Could you check a few things on this model? Use its own coordinates, in mm. A direction names the side the tool comes from. Round coordinates to 2 decimals unless told otherwise and drop trailing zeros. Loops run counter-clockwise (first coordinate to the right, second up) from the corner with the lowest first, then second, coordinate; pieces in that order, holes last. Notation, with made-up numbers: M 31,85 L 47,85 A22 ccw 47,94 Z; hole C 0,44.25 d10. An arc over 180 degrees is marked long. One line per item, written item: value. Start each with the question number.
Q1. Please list where these lines run through material, in increasing order: line 1 along Z through (x, y) = (-40, 3.7); line 2 along Y through (x, z) = (-40.5, -67.5); line 3 along Z through (x, y) = (-7.5, 29).
Q2. Which directions (+Z, -Z, +X, -X, +Y, -Y) give clear straight access to the entire face, cutting with the end or side of a thin tool? Please do faces 1 (the face through (-15, 65, -75)), 2 (the face through (-43, 7, -71)), 3 (the face through (-25, 5, -29)).
Q3. Thinking about a two-plate mould opening in Z: for faces 4 (the face through (-40.066, 41.048, -65.07)), 5 (the face through (-7, 6, -72)), 6 (the face through (-10, 2, -102)), which applies, released by +Z, released by -Z, zero draft, split by the parting line, or undercut?
Q4. Imagine slicing it at B-B (z = -10). Please give me the cut outline in (x, y).
Q5. Imagine slicing it at A-A (y = 16). Please give me the cut outline in (x, z).
Q6. I'm going to push flat-ended pins straight in: pin 1 Ø4 at (x, y) = (-8, 24) entering from +Z; pin 2 Ø5 at (x, z) = (-28.5, -50.5) entering from +Y; pin 3 Ø8 at (y, z) = (93, -75.5) entering from +X; pin 4 Ø5.5 at (x, z) = (-24, -80) entering from +Y. Where does each tip first touch, or does it pass through?
Q7. Imagine slicing it at D-D (x = -45.5). Please give me the cut outline in (y, z), then the cut area to 3 significant figures.
Q8. Imagine slicing it at C-C (x = -9.5). Please give me the cut outline in (y, z).
Autodesk Inventor part; units mm, degrees
ref_plane "YZ Plane" through (0, 0, 0) normal (1, 0, 0) x (0, 1, 0)
ref_plane "XZ Plane" through (0, 0, 0) normal (0, 1, 0) x (-1, 0, 0)
ref_plane "XY Plane" through (0, 0, 0) normal (0, 0, 1) x (1, 0, 0)
sketch "Sketch1" plane through (0, 0, 0) normal (0, 1, 0) x (-1, 0, 0)
  point P0 (0, 0)
sketch "Sketch2" plane through (0, 0, 0) normal (0, 1, 0) x (-1, 0, 0)
  line L0 (0, 0) -> (50, 0)
  line L1 (50, 0) -> (50, -110)
  line L2 (50, -110) -> (0, -110)
  line L3 (0, -110) -> (0, 0)
  line L4 (25, 0) -> (25, -110) construction
  line L5 (50, -55) -> (0, -55) construction
  circle A0 centre (40, -10) radius 2
  circle A1 centre (40, -100) radius 2
  circle A2 centre (10, -10) radius 2
  circle A3 centre (10, -100) radius 2
  dimension "d0" = 50
  dimension "d1" = 110
  dimension "d2" = 4
  dimension "d3" = 10
  dimension "d4" = 10
  dimension "d7" = 90
  dimension "d10" = 30
extrude "Extrusion1" add sketch "Sketch2" along normal blind 5
sketch "Sketch3" plane through (0, 5, 0) normal (0, 1, 0) x (1, 0, 0)
  line L0 (-50, 110) -> (-50, 0)
  line L1 (0, 60) -> (-50, 60)
  line L2 (-50, 60) -> (-50, 70)
  line L3 (0, 70) -> (0, 60)
  line L4 (-50, 0) -> (0, 0)
  line L5 (0, 110) -> (-50, 110) construction
  line L6 (0, 0) -> (0, 110)
  circle A0 centre (-25, 80) radius 3.5
  arc A1 (-15, 80) -> (-35, 80) centre (-25, 80) ccw
  line L7 (-35, 80) -> (-35, 70)
  line L8 (-15, 80) -> (-15, 70)
  line L9 (-50, 70) -> (-35, 70)
  line L10 (-15, 70) -> (0, 70)
  dimension "d15" = 60
  dimension "d17" = 7
  dimension "d18" = 30
extrude "Extrusion2" add sketch "Sketch3" along normal blind 120 contours L9 L7 A1 L8 L10 L3 L1 L0
chamfer "Chamfer1" distance 2 angle 45 1 edges at (-25, 5, -60)
chamfer "Chamfer2" distance 3 angle 45 5 edges at (-7.5, 5, -70) (-42.5, 5, -70) (-25, 5, -90) (-15, 5, -75) (-35, 5, -75)
sketch "Sketch4" plane through (0, 125, -70) normal (0, 0, -1) x (-1, 0, 0)
  line L0 (0, 0) -> (15, 0)
  line L1 (15, -117) -> (0, -117)
  line L2 (35, 0) -> (50, 0)
  line L3 (50, -117) -> (35, -117)
  circle A0 centre (9.5, -109) radius 2
  circle A1 centre (40.5, -109) radius 2
  circle A2 centre (9.5, -82) radius 2
  circle A3 centre (40.5, -82) radius 2
  line L4 (0, -117) -> (0, 0)
  line L5 (50, -117) -> (50, 0)
  line L6 (0, -120) -> (50, -120)
  point P0 (0, -125)
  dimension "d27" = 4
  dimension "d29" = 4
  dimension "d31" = 4
  dimension "d32" = 4
  dimension "d33" = 27
  dimension "d34" = 27
  dimension "d35" = 9.5
  dimension "d36" = 9.5
  dimension "d37" = 9.5
  dimension "d38" = 9.5
  dimension "d40" = 11
  dimension "d41" = 11
extrude "Extrusion3" cut sketch "Sketch4" against normal blind 10
chamfer "Chamfer3" distance 2 angle 45 8 edges at (-25, 125, -90) (-35, 125, -75) (-15, 125, -75) (-7.5, 125, -70) (0, 125, -65) (-25, 125, -60) (-42.5, 125, -70) (-50, 125, -65)
chamfer "Chamfer4" distance 3 angle 45 4 edges at (0, 2.5, -110) (-50, 2.5, -110) (0, 2.5, 0) (-50, 2.5, 0)
Report:
1. line 1: z = -110 to -102, -98 to -12, -8 to 0
1. line 2: y = 0 to 14, 18 to 41, 45 to 125
1. line 3: z = -70 to -60
2. face 1: -Z, +X, +Y
2. face 2: -Z, -X, +Y
2. face 3: +Z, +X, -X, +Y
3. face 4: zero draft
3. face 5: released by -Z
3. face 6: undercut
4. outline: M -50,0 L -42,0 L -42,5 L -50,5 Z; M -38,0 L -12,0 L -12,5 L -38,5 Z; M -8,0 L 0,0 L 0,5 L -8,5 Z
5. outline: M -50,-70 L -42.5,-70 L -42.5,-60 L -50,-60 Z; M -38.5,-70 L -35,-70 L -35,-80 A10 ccw -15,-80 L -15,-70 L -11.5,-70 L -11.5,-60 L -38.5,-60 Z; M -7.5,-70 L 0,-70 L 0,-60 L -7.5,-60 Z; hole C -25,-80 d7
6. pin 1: stops at z = -60
6. pin 2: stops at y = 5
6. pin 3: stops at x = -15
6. pin 4: stops at y = 125
7. outline: M 0,-110 L 5,-110 L 5,-73 L 8,-70 L 123,-70 L 125,-68 L 125,-62 L 123,-60 L 7,-60 L 5,-58 L 5,0 L 0,0 Z
7. area: 1,750 mm²
8. outline: M 0,-110 L 5,-110 L 5,-101.94 L 0,-101.94 Z; M 0,-98.06 L 5,-98.06 L 5,-73 L 8,-70 L 14,-70 L 14,-60 L 7,-60 L 5,-58 L 5,-11.94 L 0,-11.94 Z; M 0,-8.06 L 5,-8.06 L 5,0 L 0,0 Z; M 18,-70 L 41,-70 L 41,-60 L 18,-60 Z; M 45,-70 L 123,-70 L 125,-68 L 125,-62 L 123,-60 L 45,-60 Z
